Read the model definition and answer for the solid it produces. Units are mm, in the model's axes. A direction names the side the tool comes from. Give positions to 0.01 mm unless a question says otherwise; leave off trailing zeros. Loops run counter-clockwise (first coordinate to the right, second up) from the corner with the lowest first, then second, coordinate; pieces in that order, holes last. Notation, with made-up numbers: (-27.75, 46.25) - (-0.75, 46.25) arc R20 ccw to (-0.75, 66.25) - close; hole circle Ø8 at (-29, 62.5). An arc over 180 degrees is marked (long way). Use a Markdown table: item, result. Add a question column.
Item 1: A cutting plane is placed at A-A (x = -18.55). Determine the outline of the cut face in (y, z).
Item 2: Consider probe 1 along Z at (x, y) = (-18.55, 16.9); probe 2 along Z at (x, y) = (-10.5, 5); probe 3 along Y at (x, z) = (-1.5, 7). Determine where each line is inside the solid, lowest interval first. Write a range as [from, to].
Item 3: Each of these flat-tipped pins is pushed along its axis until it touches: P1, Ø1, axis at x = 5.5, z = 3, coming from the -Y side; P2, Ø4.5, axis at x = -18.55, z = 5.2, coming from the -Y side; P3, Ø3, axis at x = -20, z = 3, coming from the -Y side. Where does it stop, or does it pass through?
Item 4: Which of the six approach directions +Z, -Z, +X, -X, +Y, -Y give full straight-line access (tool end or side, diameter ignored) to faces 1 (the face through (-14.9, 13.2, 4.4)), 2 (the face through (-23, 17, 4)), 3 (the face through (7.8, -9.56, 7.03))?
Item 5: A cutting plane is placed at B-B (z = 1). Determine the outline of the cut face in (x, y).
Item 6: For a pull along Z with two mould halves and no side action, classify faces 4 (the face through (-16.85, 16.59, 5.27)), 5 (the face through (-7, 11, 9)), 6 (the face through (-11.8, -2.63, 7.03)) as +Z half, -Z half, draft (parallel to the pull), parting line (faces both ways), or undercut.
from build123d import *

# Parameters (mm, degrees)
F0_R     = 9.1
F1_DEPTH = 9
F2_SIZE  = 0.5
F3_R     = 1.7
F4_DEPTH = 5.0047524467
F5_R     = 9.1
F6_DEPTH = 4


# Not quite as in the source:
# - a feature names something its author has since deleted; it is built from what else it names


with BuildPart() as f1:
    # F0 (on Top) → F1 (new body)
    with BuildSketch(Plane.XY):
        with BuildLine():
            Line((-14, 11.0595270927), (-14, 5.2172651566))
            ThreePointArc((-14, 5.2172651566), (8.443285949, -12.9592956308), (0, 14.6595270927))
            ThreePointArc((0, 14.6595270927), (-1.647244668, 17.8011844795), (-4.9638694584, 19.0595270927))
            Line((-4.9638694584, 19.0595270927), (-23, 19.0595270927))
            Line((-23, 19.0595270927), (-23, 14.0595270927))
            Line((-23, 14.0595270927), (-17, 14.0595270927))
            ThreePointArc((-17, 14.0595270927), (-14.8786796564, 13.1808474363), (-14, 11.0595270927))
        make_face()
        with Locations((0, -0.4404729073)):
            Circle(F0_R, mode=Mode.SUBTRACT)
    extrude(amount=F1_DEPTH)

    # F2
    f2_edges = [f1.edges().sort_by_distance(p)[0] for p in [
        (-23, 16.559527, 0),
        (-20, 14.059527, 0),
        (-14.87868, 13.180847, 0),
        (-14, 8.138396, 0),
        (8.443286, -12.959296, 0),
        (-1.647245, 17.801184, 0),
        (-13.981935, 19.059527, 0),
        (-9.1, -0.440473, 0),
        (8.443286, -12.959296, 9),
        (-14, 8.138396, 9),
        (-20, 14.059527, 9),
        (-14.87868, 13.180847, 9),
        (-23, 16.559527, 9),
        (-13.981935, 19.059527, 9),
        (-1.647245, 17.801184, 9),
        (-23, 14.059527, 4.5),
    ]]
    chamfer(f2_edges, length=F2_SIZE)

    # F3 (on face) → F4 (cut, through all)
    with BuildSketch(Plane(origin=(0, 19.0595270927, 0), x_dir=(-1, 0, 0), z_dir=(0, 1, 0))):
        with Locations((18.55, 5.2)):
            Circle(F3_R)
    extrude(amount=-F4_DEPTH, mode=Mode.SUBTRACT)

    # F5 (on face) → F6 (cut)
    with BuildSketch(Plane.XY.offset(9)):
        Polygon((-10.4585305038, -9.5299800281), (2.6424788226, -14.0425795703), (13.1010093265, -4.9530724494), (10.4585305038, 8.6490342136), (-2.6424788226, 13.1616337557), (-13.1010093265, 4.0721266349), align=None)
        with Locations((0, -0.4404729073)):
            Circle(F5_R, mode=Mode.SUBTRACT)
    extrude(amount=-F6_DEPTH, mode=Mode.SUBTRACT)


solid = f1.part
Geometry says:
| question | item | result |
|---|---|---|
| 1 | outline | (14.06, 0.5) - (14.56, 0) - (18.56, 0) - (19.06, 0.5) - (19.06, 3.5) - (14.06, 3.5) - close; (14.06, 6.9) - (19.06, 6.9) - (19.06, 8.5) - (18.56, 9) - (14.56, 9) - (14.06, 8.5) - close |
| 2 | probe 1 | [0, 3.5], [6.9, 9] |
| 2 | probe 2 | [0, 5] |
| 2 | probe 3 | [-15.47, -12.62], [12.77, 17.67] |
| 3 | P1 | y = -14.69 |
| 3 | P2 | y = 13.98 |
| 3 | P3 | y = 14.06 |
| 4 | face 1 | +Z, -Z, -X |
| 4 | face 2 | +Z, -Z, -X, +Y, -Y |
| 4 | face 3 | +Z |
| 5 | outline | (-23, 14.56) - (-22.5, 14.06) - (-17, 14.06) arc R3 cw to (-14, 11.06) - (-14, 5.22) arc R15.1 ccw (long way) to (0, 14.66) arc R5 ccw to (-4.96, 19.06) - (-23, 19.06) - close; hole circle Ø18.2 at (0, -0.44) |
| 6 | face 4 | undercut |
| 6 | face 5 | +Z half |
| 6 | face 6 | draft |
